Geometry: final body of the model. Coordinates: model frame, mm. A direction names the side the tool comes from. Give positions to 0.01 mm unless a question says otherwise; leave off trailing zeros. Write each loop counter-clockwise with the first axis right and the second up, starting at its lowest first coordinate (ties: lowest second). Pieces come first, ordered by that corner, then holes.
Q1. Draft query along X for faces 1 (the face through (29.11, 0.57, 60.01)), 2 (the face through (25.7, -8.1, 16.5)), 3 (the face through (0, 0, 55.173)), 4 (the face through (14, 0, 60.173)). Return one class per face: pulls with the +X half, pulls with the -X half, needs draft (parallel to the pull), parting line crosses it, or undercut.
Q2. Cut plane A-A on z = 6. Return the cut outline in (x, y).
Q3. Pin query (flat end, axial travel): pin 1 (5 mm diameter, centred on y = 3.5, z = 36, fed in from -X); pin 2 (3 mm diameter, centred on x = -1, y = 13.5, fed in from +Z); pin 3 (1.4 mm diameter, centred on x = 0.5, y = -0.5, fed in from -Z). Return the tip coordinate at first contact, or that it passes through.
Q4. Line query: L1, parallel to X at y = 0, z = 3; L2, parallel to Z at x = 7.5, y = 28. Output: solid intervals per line, ascending.
Q5. Reachability of faces 5 (the face through (-3.068, -23.364, 50.726)), 6 (the face through (0, 0, 50.051)), 7 (the face through (-3.99, 0.41, 56.16)) from +Z, -Z, +X, -X, +Y, -Y: full face, straight path, thin tool, end or side. Return the list, or none.
```python
from build123d import *

# Parameters (mm, degrees)
F2_W     = 10
F2_H     = 10.684083
F3_DEPTH = 50
F4_SIZE  = 2


with BuildPart() as f1:
    # F0 (on Front) → F1 (revolve)
    with BuildSketch(Plane.XZ):
        with BuildLine():
            ThreePointArc((5.221926, 49.283396), (20.015155, 37.642235), (26.638337, 20.021517))
            Line((26.638337, 20.021517), (27.70567, 7.821847))
            Line((27.70567, 7.821847), (29.05, 7.821847))
            Line((29.05, 7.821847), (29.05, 1.821847))
            Line((29.05, 1.821847), (32.158393, 1.821847))
            ThreePointArc((32.158393, 1.821847), (32.89567, 2.146257), (33.154587, 2.909003))
            Line((33.154587, 2.909003), (31.619311, 20.457296))
            ThreePointArc((31.619311, 20.457296), (28.637021, 32.493148), (22.112054, 43.037369))
            ThreePointArc((22.112054, 43.037369), (20.965631, 47.074366), (23.298553, 50.562789))
            Line((23.298553, 50.562789), (27.557738, 53.164003))
            ThreePointArc((27.557738, 53.164003), (29.31231, 54.984743), (29.951671, 57.431135))
            Line((29.951671, 57.431135), (29.951671, 59.172666))
            Line((29.951671, 59.172666), (28.951671, 60.172666))
            Line((28.951671, 60.172666), (0, 60.172666))
            Line((0, 60.172666), (0, 50.051302))
            Line((0, 50.051302), (1.378953, 50.051302))
            ThreePointArc((1.378953, 50.051302), (3.338425, 49.857446), (5.221926, 49.283396))
        make_face()
    revolve(axis=Axis((0, 0, 55.111984), (0, 0, -1)))

    # F2 (on Front) → F3 (cut, symmetric)
    with BuildSketch(Plane.XZ):
        with Locations((0, 60.514708)):
            Rectangle(F2_W, F2_H)
    extrude(amount=F3_DEPTH, both=True, mode=Mode.SUBTRACT)

    # F4
    f4_edges = [f1.edges().sort_by_distance(p)[0] for p in [
        (-5, 0, 55.172666),
        (5, 0, 55.172666),
    ]]
    chamfer(f4_edges, length=F4_SIZE)


solid = f1.part
```
Data:
1. face 1: pulls with the +X half
1. face 2: undercut
1. face 3: undercut
1. face 4: needs draft
2. outline: circle Ø65.77 at (0, 0); hole circle Ø58.1 at (0, 0)
3. pin 1: stops at x = -28.01
3. pin 2: stops at z = 55.17
3. pin 3: stops at z = 50.05
4. L1: x = -33.15 to -29.05, 29.05 to 33.15
4. L2: z = 7.82 to 31.63, 54.48 to 60.14
5. face 5: none
5. face 6: -Z
5. face 7: +Z, +Y, -Y
